from build123d import *

# Parameters (mm, degrees)
SKETCH1_W               = 72
SKETCH1_H               = 60
BOSS_EXTRUDE1_DEPTH     = 5
SKETCH2_W               = 5
SKETCH2_H               = 60
BOSS_EXTRUDE2_DEPTH     = 70
SKETCH3_W               = 5
SKETCH3_H               = 60
BOSS_EXTRUDE3_DEPTH     = 70
BOSS_EXTRUDE4_DEPTH     = 60
CHAMFER1_SIZE           = 42
CHAMFER1_SIZE_2         = 35.242184509
CHAMFER2_SIZE           = 15.000718891
CHAMFER2_SIZE_2         = 50
SKETCH12_W              = 20.2
SKETCH12_H              = 20.2
CUT_EXTRUDE8_DEPTH      = 67
CUT_EXTRUDE1_DEPTH      = 117.978630527
CUT_EXTRUDE1_DEPTH_BACK = 117.978630527
SKETCH5_R               = 16.5
SKETCH6_R               = 1.65
CUT_EXTRUDE2_DEPTH      = 121.037494142
SKETCH7_R               = 4
CUT_EXTRUDE4_DEPTH      = 117.978630527
CUT_EXTRUDE5_DEPTH      = 105.748460609
CUT_EXTRUDE5_DEPTH_BACK = 105.748460609
SKETCH8_R               = 2.65
CUT_EXTRUDE6_DEPTH      = 121.037494142
CUT_EXTRUDE6_DEPTH_BACK = 121.037494142
SKETCH9_R               = 2.65
FILLET1_R               = 5
SKETCH10_R              = 2.65
CUT_EXTRUDE7_DEPTH      = 10
CUT_EXTRUDE9_DEPTH      = 121.037494142
CUT_EXTRUDE9_DEPTH_BACK = 121.037494142
CUT_EXTRUDE10_REACH     = 122.037
SKETCH14_W              = 12
SKETCH14_H              = 8


with BuildPart() as part:
    # Sketch1 → Boss-Extrude1 (new body)
    with BuildSketch(Plane(origin=(0, 0, 0), x_dir=(1, 0, 0), z_dir=(0, 1, 0))):
        with Locations((36, 30)):
            Rectangle(SKETCH1_W, SKETCH1_H)
    extrude(amount=BOSS_EXTRUDE1_DEPTH)

    # Sketch2 → Boss-Extrude2 (add)
    with BuildSketch(Plane(origin=(0, 5, 0), x_dir=(1, 0, 0), z_dir=(0, 1, 0))):
        with Locations((2.5, 30)):
            Rectangle(SKETCH2_W, SKETCH2_H)
    extrude(amount=BOSS_EXTRUDE2_DEPTH)

    # Sketch3 → Boss-Extrude3 (add)
    with BuildSketch(Plane(origin=(0, 5, 0), x_dir=(1, 0, 0), z_dir=(0, 1, 0))):
        with Locations((27.7, 30)):
            Rectangle(SKETCH3_W, SKETCH3_H)
    extrude(amount=BOSS_EXTRUDE3_DEPTH)

    # Sketch11 → Boss-Extrude4 (add)
    with BuildSketch(Plane(origin=(0, 0, -60), x_dir=(-1, 0, 0), z_dir=(0, 0, -1))):
        Polygon((-25.2, 25), (-15.1, 35.1), (-5, 25), (-5, 75), (-25.2, 75), align=None)
    extrude(amount=-BOSS_EXTRUDE4_DEPTH)

    # Chamfer1
    # the kernel refuses this chamfer: 42, 35.242184509 mm, written as the material it adds along each edge
    with BuildSketch(Plane(origin=(30.2, 5, -60), x_dir=(0.9996889667359942, -0.02493932209023436, 0), z_dir=(0, 0, 1))) as chamfer1_piece_1_section:
        Polygon((CHAMFER1_SIZE * 0.999688966736, CHAMFER1_SIZE * 0.0249393220902), (-CHAMFER1_SIZE_2 * 0.0249393220905, CHAMFER1_SIZE_2 * 0.999688966749), (0, 0), align=None)
    chamfer1_piece_1 = extrude(amount=60, mode=Mode.PRIVATE)
    chamfer1_piece_1 = split(chamfer1_piece_1, bisect_by=Plane(origin=(72, 16.573415306, -30), z_dir=(-1, 0, 0)), keep=Keep.TOP, mode=Mode.PRIVATE)
    add(chamfer1_piece_1)

    # Chamfer2
    # the kernel refuses this chamfer: 50, 15.000718891 mm, written as the material it takes off along each edge
    with BuildSketch(Plane(origin=(159.997065138, 75, -60), x_dir=(0, 0.12207157319780576, 0.9925213000318999), z_dir=(-1, 0, 0))) as chamfer2_piece_1:
        Polygon((CHAMFER2_SIZE * 0.99252130002, -CHAMFER2_SIZE * 0.122071573196), (-CHAMFER2_SIZE_2 * 0.122071573198, -CHAMFER2_SIZE_2 * 0.992521300032), (0, 0), align=None)
    extrude(amount=289.794130277, mode=Mode.SUBTRACT)
    with BuildSketch(Plane(origin=(159.997065138, 75, 0), x_dir=(0, 0.12207157319780576, -0.9925213000318999), z_dir=(-1, 0, 0))) as chamfer2_piece_2:
        Polygon((CHAMFER2_SIZE * 0.99252130002, CHAMFER2_SIZE * 0.122071573196), (-CHAMFER2_SIZE_2 * 0.122071573198, CHAMFER2_SIZE_2 * 0.992521300032), (0, 0), align=None)
    extrude(amount=289.794130277, mode=Mode.SUBTRACT)

    # Sketch12 → Cut-Extrude8 (cut)
    with BuildSketch(Plane(origin=(0, 75, 0), x_dir=(1, 0, 0), z_dir=(0, 1, 0))):
        with Locations((15.1, 30)):
            Rectangle(SKETCH12_W, SKETCH12_H)
    extrude(amount=-CUT_EXTRUDE8_DEPTH, mode=Mode.SUBTRACT)

    # Sketch5 → Cut-Extrude1 (cut, two sides: drawn at the far end of the back side and taken through both)
    with BuildSketch(Plane(origin=(0, 5, 0), x_dir=(1, 0, 0), z_dir=(0, 1, 0)).offset(-CUT_EXTRUDE1_DEPTH_BACK)):
        with Locations(Location((51, 30, 0), (0, 0, 270))):
            Circle(SKETCH5_R)
    extrude(amount=CUT_EXTRUDE1_DEPTH + CUT_EXTRUDE1_DEPTH_BACK, mode=Mode.SUBTRACT)

    # Sketch6 → Cut-Extrude2 (cut, through all)
    with BuildSketch(Plane.XZ):
        with Locations(Location((66.5, -14.5, 0), (0, 0, 270))):
            Circle(SKETCH6_R)
        with Locations(Location((66.5, -45.5, 0), (0, 0, 270))):
            Circle(SKETCH6_R)
        with Locations(Location((35.5, -45.5, 0), (0, 0, 270))):
            Circle(SKETCH6_R)
        with Locations(Location((35.5, -14.5, 0), (0, 0, 270))):
            Circle(SKETCH6_R)
    extrude(amount=-CUT_EXTRUDE2_DEPTH, mode=Mode.SUBTRACT)

    # Sketch7 → Cut-Extrude4 (cut, through all)
    with BuildSketch(Plane(origin=(0, 5, 0), x_dir=(1, 0, 0), z_dir=(0, 1, 0))):
        with Locations((66.5, 45.5)):
            Circle(SKETCH7_R)
        with Locations((66.5, 14.5)):
            Circle(SKETCH7_R)
        with Locations((35.5, 14.5)):
            Circle(SKETCH7_R)
        with Locations((35.5, 45.5)):
            Circle(SKETCH7_R)
    extrude(amount=CUT_EXTRUDE4_DEPTH, mode=Mode.SUBTRACT)

    # Sketch8 → Cut-Extrude5 (cut, two sides: drawn at the far end of the back side and taken through both)
    with BuildSketch(Plane(origin=(30.2, 0, 0), x_dir=(0, 0, -1), z_dir=(1, 0, 0)).offset(-CUT_EXTRUDE5_DEPTH_BACK)):
        with Locations((30, 65)):
            Circle(SKETCH8_R)
    extrude(amount=CUT_EXTRUDE5_DEPTH + CUT_EXTRUDE5_DEPTH_BACK, mode=Mode.SUBTRACT)

    # Sketch9 → Cut-Extrude6 (cut, two sides: drawn at the far end of the back side and taken through both)
    with BuildSketch(Plane.XZ.offset(-CUT_EXTRUDE6_DEPTH_BACK)):
        with Locations(Location((15, -30, 0), (0, 0, 270))):
            Circle(SKETCH9_R)
    extrude(amount=CUT_EXTRUDE6_DEPTH + CUT_EXTRUDE6_DEPTH_BACK, mode=Mode.SUBTRACT)

    # Fillet1
    fillet1_edges = [part.edges().sort_by_distance(p)[0] for p in [
        (72, 2.583909963, -60),
        (72, 2.583909963, 0),
    ]]
    fillet(fillet1_edges, radius=FILLET1_R)

    # Sketch10 → Cut-Extrude7 (cut)
    with BuildSketch(Plane.ZY):
        with Locations((-30, 15)):
            Circle(SKETCH10_R)
    extrude(amount=-CUT_EXTRUDE7_DEPTH, mode=Mode.SUBTRACT)

    # Sketch13 → Cut-Extrude9 (cut, two sides: drawn at the far end of the back side and taken through both)
    with BuildSketch(Plane.XY.offset(-CUT_EXTRUDE9_DEPTH_BACK)):
        Polygon((5, 5), (4, 5), (5, 9), align=None)
        Polygon((25.2, 5), (26.2, 5), (25.2, 9), align=None)
    extrude(amount=CUT_EXTRUDE9_DEPTH + CUT_EXTRUDE9_DEPTH_BACK, mode=Mode.SUBTRACT)

    # Cut-Extrude10: up to this face of the body (flat: up to its plane)
    cut_extrude10_end = Plane(part.part.faces().sort_by_distance((15.1, 5, -59.366909169))[0])
    # Sketch14 → Cut-Extrude10 (cut, up to the picked face)
    with BuildSketch(Plane(origin=(0, 75, 0), x_dir=(1, 0, 0), z_dir=(0, 1, 0)), mode=Mode.PRIVATE) as cut_extrude10_sk1:
        with Locations((15.1, 44.1)):
            Rectangle(SKETCH14_W, SKETCH14_H)
    cut_extrude10_tool1 = split(extrude(cut_extrude10_sk1.sketch, amount=-CUT_EXTRUDE10_REACH, mode=Mode.PRIVATE), bisect_by=cut_extrude10_end, keep=Keep.BOTH, mode=Mode.PRIVATE)
    # Sketch14 → Cut-Extrude10 (cut, up to the picked face)
    with BuildSketch(Plane(origin=(0, 75, 0), x_dir=(1, 0, 0), z_dir=(0, 1, 0)), mode=Mode.PRIVATE) as cut_extrude10_sk2:
        with Locations((15.1, 15.9)):
            Rectangle(SKETCH14_W, SKETCH14_H)
    cut_extrude10_tool2 = split(extrude(cut_extrude10_sk2.sketch, amount=-CUT_EXTRUDE10_REACH, mode=Mode.PRIVATE), bisect_by=cut_extrude10_end, keep=Keep.BOTH, mode=Mode.PRIVATE)
    add(cut_extrude10_tool1.solids().sort_by(Axis((15.1, 75, -44.1), (0, -1, 0)))[0], mode=Mode.SUBTRACT)
    add(cut_extrude10_tool2.solids().sort_by(Axis((15.1, 75, -15.9), (0, -1, 0)))[0], mode=Mode.SUBTRACT)


solid = part.part
Part model, mm, in its own coordinate system. A direction names the side the tool comes from. Give positions to 0.01 mm unless a question says otherwise; leave off trailing zeros. Loops run counter-clockwise (first coordinate to the right, second up) from the corner with the lowest first, then second, coordinate; pieces in that order, holes last.
(1) Pin check, flat tips, straight feed: pin 1 (5 mm diameter, centred on x = 59, z = -10.5, fed in from +Y); pin 2 (6.5 mm diameter, centred on y = 47, z = -15, fed in from +X); pin 3 (6 mm diameter, centred on x = 12.5, y = 53.5, fed in from -Z). Stop position of each tip, or through.
Return value:
pin 1: stops at y = 18.17
pin 2: stops at x = 30.2
pin 3: stops at z = -52.35
(2) 3-axis set-ups, long thin cutter, end or side, ignore diameter. For faces 1 (the flat face through (23, 50, -40.1)), 2 (the cylindrical face through (70, 4, -1)), 3 (the flat face through (5, 34, -30)), 4 (the flat face through (9, 29, -50)), 5 (the flat face through (33, 12, -60)): which of +Z, -Z, +X, -X, +Y, -Y reach the whole face in a straight line?
Return value:
face 1: +Y
face 2: +Z, +X, +Y, -Y
face 3: none
face 4: +Z, -Z
face 5: -Z, +X, -X, +Y, -Y
(3) Band-saw the part on C-C (x = 41.5). Write the cut outline in (y, z).
Return value:
outline: (0, -60) - (25, -60) - (30.76, -58.27) - (30.76, -43.49) - (0, -43.49) - close; (0, -16.51) - (30.76, -16.51) - (30.76, -1.73) - (25, 0) - (0, 0) - close
(4) Band-saw the part on B-B (z = -30). Count the separate pieces of the cut face and the enclosed holes in it, and give its area (3 significant figures).
Return value:
separate pieces: 6
enclosed holes: 0
area: 938 mm2
(5) Band-saw the part on A-A (y = 15). Write the cut outline in (x, z), and give its area (3 significant figures).
Return value:
outline: (0, -60) - (5, -60) - (5, -32.65) - (0, -32.65) - close; (0, -27.35) - (5, -27.35) - (5, 0) - (0, 0) - close; (25.2, -60) - (60.28, -60) - (60.28, -43.64) arc R16.5 cw (long way) to (60.28, -16.36) - (60.28, 0) - (25.2, 0) - close; hole circle Ø8 at (35.5, -45.5); hole circle Ø8 at (35.5, -14.5)
area: 1,560 mm2
(6) Band-saw the part on D-D (z = -21.5). Write the cut outline in (x, y).
Return value:
outline: (0, 0) - (36.86, 0) - (36.86, 34.66) - (30.2, 40.24) - (30.2, 75) - (25.2, 75) - (25.2, 9) - (26.2, 5) - (4, 5) - (5, 9) - (5, 75) - (0, 75) - close; (65.14, 0) - (72, 0) - (72, 5.17) - (65.14, 10.92) - close
(7) Pull direction X, two halves, no side cores. Call faces 6 (the flat face through (3, 75, -30)), 7 (the flat face through (30.2, 57, -30)), 8 (the flat face through (15, 47, -11.9)): pulls with the +X half, pulls with the -X half, needs draft (parallel to the pull), parting line crosses it, or undercut.
Return value:
face 6: needs draft
face 7: pulls with the +X half
face 8: undercut
(8) Drill centre lines: line 1 along X through (y, z) = (2.9, -30); line 2 along Y through (x, z) = (2.75, -30); line 3 along Z through (x, y) = (51, 17). Where is each one in solid material? Low to high.
Return value:
line 1: x = 0 to 12.35, 17.65 to 34.5, 67.5 to 72
line 2: y = 0 to 12.35, 17.65 to 62.35, 67.65 to 75
line 3: z = -60 to -46.5, -13.5 to 0
